Work out the finished part from the listing and answer in its coordinate system (mm). A direction names the side the tool comes from. Give positions to 0.01 mm unless a question says otherwise; leave off trailing zeros. Loops run counter-clockwise (first coordinate to the right, second up) from the corner with the lowest first, then second, coordinate; pieces in that order, holes last. Notation, with made-up numbers: (17, 37) -> (74, 37) arc R34 ccw to (74, 73) -> close; hole circle Ø3 at (-31.5, 43). An arc over 180 degrees is marked (long way). Answer as CSV lines item,"result". Start each with the question number.
1. Find section B-B, the plane z = -43. Give the vertices of the cut face in (x, y).
2. Find section C-C, the plane y = 10.5. Give the vertices of the cut face in (x, z).
3. Find the intervals of material crossed by line 1 along Y through (x, z) = (7, 47); line 2 along X through (y, z) = (8.5, -11.5); line 3 along Y through (x, z) = (-23, 51), in increasing order.
4. Flat-ended cylindrical pins translate along their axes: pin 1 Ø4 at (y, z) = (6, -16.5) entering from -X; pin 2 Ø10 at (x, z) = (-21.5, 37) entering from +Y; pin 3 Ø6 at (y, z) = (7.5, 30.5) entering from +X. Find the tip coordinate at first contact, or state that the pin passes through.
5. A tool of negligible diameter and unlimited length cuts with its end or side. For faces 4 (the face through (0, 0, 1)), 5 (the face through (19, 1, 1)), 6 (the face through (0.1, 0.8, 75)), 7 (the face through (0, 12.7, 1)), 8 (the face through (-12.7, 7, 1)), from which of +Z, -Z, +X, -X, +Y, -Y can it reach the whole face along a straight path? Write none if from no direction.
6. Find section D-D, the plane x = -19.5. Give the vertices of the cut face in (y, z), and give its area (3 significant figures).
7. Find section A-A, the plane x = 1.5. Give the vertices of the cut face in (y, z).
8. Determine the mould class of faces 1 (the face through (12.7, 7, 1)), 2 (the face through (-11.7, 7, 1)), 3 (the face through (0.1, 0.8, -75)) for opening direction X: +X half, -X half, draft (parallel to the pull), parting line (faces both ways), or undercut.
from build123d import *

# Parameters (mm, degrees)
SALIENTE_EXTRUIR1_DEPTH = 75


with BuildPart() as part:
    # Croquis1 → Saliente-Extruir1 (new body, symmetric)
    with BuildSketch(Plane.XY):
        Polygon((0, 13.7), (12.7, 13.7), (12.7, 1), (25.4, 1), (25.4, 0), (-25.4, 0), (-25.4, 1), (-12.7, 1), (-12.7, 13.7), align=None)
        Polygon((0, 12.7), (-11.7, 12.7), (-11.7, 1), (11.7, 1), (11.7, 12.7), align=None, mode=Mode.SUBTRACT)
    extrude(amount=SALIENTE_EXTRUIR1_DEPTH, both=True)


solid = part.part
Resolved:
1,outline,"(-25.4, 0) -> (25.4, 0) -> (25.4, 1) -> (12.7, 1) -> (12.7, 13.7) -> (-12.7, 13.7) -> (-12.7, 1) -> (-25.4, 1) -> close; hole (-11.7, 1) -> (11.7, 1) -> (11.7, 12.7) -> (-11.7, 12.7) -> close"
2,outline,"(-12.7, -75) -> (-11.7, -75) -> (-11.7, 75) -> (-12.7, 75) -> close; (11.7, -75) -> (12.7, -75) -> (12.7, 75) -> (11.7, 75) -> close"
3,line 1,"y = 0 to 1, 12.7 to 13.7"
3,line 2,"x = -12.7 to -11.7, 11.7 to 12.7"
3,line 3,"y = 0 to 1"
4,pin 1,"stops at x = -12.7"
4,pin 2,"stops at y = 1"
4,pin 3,"stops at x = 12.7"
5,face 4,"+Z, -Z, +X, -X, -Y"
5,face 5,"+Z, -Z, +X, +Y"
5,face 6,"+Z, +X, -X, +Y, -Y"
5,face 7,"+Z, -Z"
5,face 8,"+Z, -Z, -X, +Y"
6,outline,"(0, -75) -> (1, -75) -> (1, 75) -> (0, 75) -> close"
6,area,"150 mm^2"
7,outline,"(0, -75) -> (1, -75) -> (1, 75) -> (0, 75) -> close; (12.7, -75) -> (13.7, -75) -> (13.7, 75) -> (12.7, 75) -> close"
8,face 1,"+X half"
8,face 2,"undercut"
8,face 3,"draft"
